Design review of the part built by this model. Coordinates are the model's own, in mm. A direction names the side the tool comes from. Give positions to 0.01 mm unless a question says otherwise; leave off trailing zeros. Loops run counter-clockwise (first coordinate to the right, second up) from the corner with the lowest first, then second, coordinate; pieces in that order, holes last. Notation, with made-up numbers: (-21, -8.75) - (23, -8.75) arc R14 cw to (23, -0.75) - close; hole circle Ø3 at (33.25, 43.25). An arc over 180 degrees is marked (long way). Put each result on its own line as item: value. Start each with the question number.
```python
from build123d import *

# Parameters (mm, degrees)
SKETCH_1_W               = 0.64
SKETCH_1_H               = 0.64
EXTRUDE_1_DEPTH          = 8.5
EXTRUDE_1_DEPTH_BACK     = 3
CHAMFER_1_SIZE           = 0.15
CHAMFER_1_SIZE2          = 0.412121613
CHAMFER_1_PART_2_SIZE    = 0.15
CHAMFER_1_PART_2_SIZE2   = 0.412121613
PATTERN_LINEAR_1_COUNT   = 3
PATTERN_LINEAR_1_PITCH   = 2.54
PATTERN_LINEAR_1_2_COUNT = 2
PATTERN_LINEAR_1_2_PITCH = 2.54
SKETCH_2_W               = 13.02
SKETCH_2_H               = 6.9
SKETCH_2_W_2             = 0.64
SKETCH_2_H_2             = 0.64
SKETCH_2_W_3             = 5
SKETCH_2_H_3             = 1.1
EXTRUDE_2_DEPTH          = 1
EXTRUDE_3_DEPTH          = 9
SKETCH_3_W               = 1.1
SKETCH_3_H               = 3.5
CUT_EXTRUDE_2_DEPTH      = 7


with BuildPart() as part:
    # Sketch 1 → Extrude 1 (new body, two sides)
    with BuildSketch(Plane(origin=(0, 0, 0), x_dir=(1, 0, 0), z_dir=(0, 1, 0))) as extrude_1_sk:
        Rectangle(SKETCH_1_W, SKETCH_1_H)
    extrude(amount=EXTRUDE_1_DEPTH)
    extrude(extrude_1_sk.sketch, amount=-EXTRUDE_1_DEPTH_BACK)

    # Chamfer 1
    chamfer_1_edges = [part.edges().sort_by_distance(p)[0] for p in [
        (0.32, -3, 0),
        (0, -3, 0.32),
        (-0.32, -3, 0),
        (0, -3, -0.32),
    ]]
    chamfer_1_side = [part.faces().sort_by_distance(p)[0] for p in [
        (0, -3, 0),
    ]]
    chamfer(chamfer_1_edges, length=CHAMFER_1_SIZE, length2=CHAMFER_1_SIZE2, reference=chamfer_1_side[0])

    # Chamfer 1 part 2
    chamfer_1_part_2_edges = [part.edges().sort_by_distance(p)[0] for p in [
        (-0.32, 8.5, 0),
        (0, 8.5, -0.32),
        (0, 8.5, 0.32),
        (0.32, 8.5, 0),
    ]]
    chamfer_1_part_2_side = [part.faces().sort_by_distance(p)[0] for p in [
        (0, 8.5, 0),
    ]]
    chamfer(chamfer_1_part_2_edges, length=CHAMFER_1_PART_2_SIZE, length2=CHAMFER_1_PART_2_SIZE2, reference=chamfer_1_part_2_side[0])


with BuildPart() as pattern_linear_1_1:
    # Pattern Linear 1: pattern copy
    add(part.part.moved(Location(Vector(1, 0, 0) * (1 * PATTERN_LINEAR_1_PITCH))))


with BuildPart() as pattern_linear_1_2:
    # Pattern Linear 1: pattern copy
    add(part.part.moved(Location(Vector(1, 0, 0) * (2 * PATTERN_LINEAR_1_PITCH))))


with BuildPart() as pattern_linear_1_2_1:
    # Pattern Linear 1 2: pattern copy
    add(part.part.moved(Location(Vector(0, 0, 1) * (1 * PATTERN_LINEAR_1_2_PITCH))))


with BuildPart() as pattern_linear_1_2_2:
    # Pattern Linear 1 2: pattern copy
    add(pattern_linear_1_1.part.moved(Location(Vector(0, 0, 1) * (1 * PATTERN_LINEAR_1_2_PITCH))))


with BuildPart() as pattern_linear_1_2_3:
    # Pattern Linear 1 2: pattern copy
    add(pattern_linear_1_2.part.moved(Location(Vector(0, 0, 1) * (1 * PATTERN_LINEAR_1_2_PITCH))))


with BuildPart() as part_1:
    add(part.part)

    add(pattern_linear_1_1.part)  # Extrude 2 merges Pattern Linear 1_1

    add(pattern_linear_1_2.part)  # Extrude 2 merges Pattern Linear 1_2

    add(pattern_linear_1_2_1.part)  # Extrude 2 merges Pattern Linear 1 2_1

    add(pattern_linear_1_2_2.part)  # Extrude 2 merges Pattern Linear 1 2_2

    add(pattern_linear_1_2_3.part)  # Extrude 2 merges Pattern Linear 1 2_3
    # Sketch 2 → Extrude 2 (add)
    with BuildSketch(Plane(origin=(0, 0, 0), x_dir=(1, 0, 0), z_dir=(0, 1, 0))):
        with Locations((2.54, -1.259333449)):
            Rectangle(SKETCH_2_W, SKETCH_2_H)
        with Locations((0, -2.54)):
            Rectangle(SKETCH_2_W_2, SKETCH_2_H_2, mode=Mode.SUBTRACT)
        with Locations((5.08, -2.54)):
            Rectangle(SKETCH_2_W_2, SKETCH_2_H_2, mode=Mode.SUBTRACT)
        with Locations((2.54, -2.54)):
            Rectangle(SKETCH_2_W_2, SKETCH_2_H_2, mode=Mode.SUBTRACT)
        with Locations((5.08, 0)):
            Rectangle(SKETCH_2_W_2, SKETCH_2_H_2, mode=Mode.SUBTRACT)
        with Locations((2.54, 0)):
            Rectangle(SKETCH_2_W_2, SKETCH_2_H_2, mode=Mode.SUBTRACT)
        Rectangle(SKETCH_2_W_2, SKETCH_2_H_2, mode=Mode.SUBTRACT)
        with Locations((2.54, 2.740666551)):
            Rectangle(SKETCH_2_W_3, SKETCH_2_H_3)
    extrude(amount=EXTRUDE_2_DEPTH)

    # Sketch 2_3 → Extrude 3 (add)
    with BuildSketch(Plane(origin=(0, 0, 0), x_dir=(1, 0, 0), z_dir=(0, 1, 0))):
        Polygon((-5.07, 3.290666551), (-5.07, -5.809333449), (10.15, -5.809333449), (10.15, 3.290666551), (5.04, 3.290666551), (5.04, 2.190666551), (9.05, 2.190666551), (9.05, -4.709333449), (-3.97, -4.709333449), (-3.97, 2.190666551), (0.04, 2.190666551), (0.04, 3.290666551), align=None)
    extrude(amount=EXTRUDE_3_DEPTH)

    # Sketch 3 → Cut-Extrude 2 (cut)
    with BuildSketch(Plane.XZ):
        with Locations((-4.52, 1.259333449)):
            Rectangle(SKETCH_3_W, SKETCH_3_H)
        with Locations((9.6, 1.259333449)):
            Rectangle(SKETCH_3_W, SKETCH_3_H)
    extrude(amount=-CUT_EXTRUDE_2_DEPTH, mode=Mode.SUBTRACT)


solid = part_1.part
```
Item 1: Consider section D-D (z = -2). State the section outline as (x, y) points.
Item 2: For P1, Ø0.5, axis at y = -1, z = 0, coming from the -X side; P2, Ø0.5, axis at x = 5, y = -0.5, coming from the -Z side; P3, Ø0.5, axis at y = -1, z = 2.5, coming from the +X side, all flat-tipped, find the tip position at first contact; note any pin that passes through.
Item 3: Mouldability with a two-part tool opening along Z and no side actions: class faces 1 (the flat face through (2, 1, 1)), 2 (the flat face through (10.15, 4.4, 3.3)), 3 (the flat face through (2, 4, 5.809)) as pulls with the +Z half, pulls with the -Z half, needs draft (parallel to the pull), parting line crosses it, or undercut.
Item 4: Consider section A-A (y = -1.25). State the section outline as (x, z) points, plus the area to 3 significant figures.
Item 5: Machinability: for faces 4 (the flat face through (10, 7, 1)), 5 (the flat face through (5.04, 5, -3)), 6 (the flat face through (-2, 5, -2.191)), which of the approach directions +Z, -Z, +X, -X, +Y, -Y give a long, thin tool a straight path to every point of the face, cutting with its end or side? Answer none if there is none.
Item 6: Consider section B-B (z = 1.25). State the section outline as (x, y) points, plus the area to 3 significant figures.
Item 7: Consider section C-C (x = -3). State the section outline as (y, z) points, plus the area to 3 significant figures.
Item 8: For L1, parallel to Z at x = 2.5, y = 2; L2, parallel to Z at x = -0.75, y = 2.5; L3, parallel to X at y = 4, z = -2, list the stretches that pass through material, from the lowest coordinate up. Write a range as from..to.
Geometry says:
1. outline: (-5.07, 0) - (10.15, 0) - (10.15, 9) - (9.05, 9) - (9.05, 1) - (-3.97, 1) - (-3.97, 9) - (-5.07, 9) - close
2. P1: stops at x = -0.32
2. P2: stops at z = -0.32
2. P3: stops at x = 5.4
3. face 1: undercut
3. face 2: needs draft
3. face 3: pulls with the +Z half
4. outline: (-0.32, -0.32) - (0.32, -0.32) - (0.32, 0.32) - (-0.32, 0.32) - close; (-0.32, 2.22) - (0.32, 2.22) - (0.32, 2.86) - (-0.32, 2.86) - close; (2.22, -0.32) - (2.86, -0.32) - (2.86, 0.32) - (2.22, 0.32) - close; (2.22, 2.22) - (2.86, 2.22) - (2.86, 2.86) - (2.22, 2.86) - close; (4.76, -0.32) - (5.4, -0.32) - (5.4, 0.32) - (4.76, 0.32) - close; (4.76, 2.22) - (5.4, 2.22) - (5.4, 2.86) - (4.76, 2.86) - close
4. area: 2.46 mm2
5. face 4: +X, -Y
5. face 5: -Z, +Y
5. face 6: +Y
6. outline: (-5.07, 7) - (-3.97, 7) - (-3.97, 9) - (-5.07, 9) - close; (-3.97, 0) - (9.05, 0) - (9.05, 1) - (-3.97, 1) - close; (9.05, 7) - (10.15, 7) - (10.15, 9) - (9.05, 9) - close
6. area: 17.4 mm2
7. outline: (0, -3.29) - (9, -3.29) - (9, -2.19) - (1, -2.19) - (1, 4.71) - (9, 4.71) - (9, 5.81) - (0, 5.81) - close
7. area: 26.7 mm2
8. L1: z = -0.32..0.32, 2.22..2.86, 4.71..5.81
8. L2: z = -3.29..-2.19, 4.71..5.81
8. L3: x = -5.07..-3.97, 9.05..10.15
